The model under review builds one solid part; all positions refer to its coordinate system, in mm. A direction names the side the tool comes from. Coordinates: 2 decimals unless noted, no trailing zeros. Order: outer loops, then holes, each group sorted by start corner. A loop starts at its lowest first (then second) coordinate and runs counter-clockwise, first axis right, second up. Notation, with made-up numbers: M 44,61 L 98,61 A34 ccw 98,100 Z; hole C 50.25,74.5 d9. An arc over 180 degrees is marked long. Answer as CSV lines item,"result". Start each with the question number.
Q1. Wall thickness on L1, parallel to X at y = 0.5, z = 4.5; L2, parallel to X at y = 3, z = 5.75; L3, parallel to Y at x = 21, z = 0.5: over which ranges is each line inside the solid? List them lowest first. Write a range as [from, to].
Q2. Consider section C-C on z = 8.5. Write out the cut boundary in (x, y) (3 decimals), and give its area (3 significant figures).
Q3. Consider section D-D on x = 28. Write out the cut boundary in (y, z), and give its area (3 significant figures).
Q4. Machinability: for faces 1 (the face through (14, -7, 0)), 2 (the face through (9.48, 9.38, 5.07)), which of the approach directions +Z, -Z, +X, -X, +Y, -Y give a long, thin tool a straight path to every point of the face, cutting with its end or side? Answer none if there is none.
Q5. For P1, Ø6, axis at y = 24.5, z = 2.5, coming from the -X side; P2, Ø5, axis at x = 14, z = 1.5, coming from the +Y side; P3, Ø1.5, axis at y = -8.5, z = 7, coming from the +X side, all flat-tipped, find the tip position at first contact; note any pin that passes through.
Q6. The part is to be moulded in two halves that separate along X. For faces 3 (the face through (14, -7, 10)), 4 (the face through (-5.103, -17, 5)), 5 (the face through (31.8, 10, 4.9)), say which applies: +X half, -X half, draft (parallel to the pull), parting line (faces both ways), or undercut.
Q7. Consider section A-A on x = 0. Write out the cut boundary in (y, z) (3 decimals).
from build123d import *

# Parameters (mm, degrees)
F0_R            = 33.335
F1_DEPTH        = 10
F2_R            = 13.335
F3_DEPTH        = 10
F5_DEPTH        = 10
F5_COPIES_COUNT = 4


# Not quite as in the source:
# - a pattern or mirror of a feature is missing from the dataset's text; its kind, count and spacing are read off the source's solid


with BuildPart() as f1:
    # F0 (on Top) → F1 (new body)
    with BuildSketch(Plane.XY):
        Circle(F0_R)
    extrude(amount=F1_DEPTH)

    # F2 (on face) → F3 (cut, through all)
    with BuildSketch(Plane.XY.offset(10)):
        Circle(F2_R)
    extrude(amount=-F3_DEPTH, mode=Mode.SUBTRACT)

    # F4 (on Top) → F5 (cut, through all)
    with BuildSketch(Plane.XY):
        with BuildLine():
            Line((22.7701726623, 5.1030835706), (12.319933566, 5.1030835706))
            ThreePointArc((12.319933566, 5.1030835706), (13.335, 0), (12.319933566, -5.1030835706))
            Line((12.319933566, -5.1030835706), (22.7701726623, -5.1030835706))
            ThreePointArc((22.7701726623, -5.1030835706), (23.335, 0), (22.7701726623, 5.1030835706))
        make_face()
    f5 = extrude(amount=F5_DEPTH, mode=Mode.SUBTRACT)

    # F5_copies: F5 ×4 about axis
    f5_copies_axis = Axis((0, 0, 0), (0, 0, 1))
    for i in range(1, F5_COPIES_COUNT):
        add(f5.rotate(f5_copies_axis, i * 360 / F5_COPIES_COUNT), mode=Mode.SUBTRACT)


solid = f1.part
Evaluation:
1,L1,"x = [-33.33, -23.33], [23.33, 33.33]"
1,L2,"x = [-33.2, -23.14], [23.14, 33.2]"
1,L3,"y = [-25.89, -5.1], [5.1, 25.89]"
2,outline,"C 0,0 d66.67; hole M -22.77,-5.103 L -12.32,-5.103 A13.335 ccw -5.103,-12.32 L -5.103,-22.77 A23.335 ccw 5.103,-22.77 L 5.103,-12.32 A13.335 ccw 12.32,-5.103 L 22.77,-5.103 A23.335 ccw 22.77,5.103 L 12.32,5.103 A13.335 ccw 5.103,12.32 L 5.103,22.77 A23.335 ccw -5.103,22.77 L -5.103,12.32 A13.335 ccw -12.32,5.103 L -22.77,5.103 A23.335 ccw Z"
2,area,"2,520 mm²"
3,outline,"M -18.09,0 L 18.09,0 L 18.09,10 L -18.09,10 Z"
3,area,"362 mm²"
4,face 1,"-Z, +X, -X, +Y, -Y"
4,face 2,"+Z, -Z"
5,P1,"stops at x = -25.47"
5,P2,"stops at y = 31.29"
5,P3,"stops at x = 32.42"
6,face 3,"draft"
6,face 4,"undercut"
6,face 5,"parting line"
7,outline,"M -33.335,0 L -23.335,0 L -23.335,10 L -33.335,10 Z; M 23.335,0 L 33.335,0 L 33.335,10 L 23.335,10 Z"
